```python
from build123d import *

# Parameters (mm, degrees)
SKETCH_W     = 50
SKETCH_H     = 50
PAD_DEPTH    = 50
SKETCH001_W  = 45
SKETCH001_H  = 45
POCKET_DEPTH = 45
FILLET_R     = 2
FILLET001_R  = 2
FILLET002_R  = 2
FILLET003_R  = 2


with BuildPart() as part:
    # Sketch → Pad (new body)
    with BuildSketch(Plane.XY):
        Rectangle(SKETCH_W, SKETCH_H)
    extrude(amount=PAD_DEPTH)

    # Sketch001 (on Face6 of Pad) → Pocket (cut)
    with BuildSketch(Plane.XY.offset(50)):
        Rectangle(SKETCH001_W, SKETCH001_H)
    extrude(amount=-POCKET_DEPTH, mode=Mode.SUBTRACT)

    # Fillet
    fillet_edges = [part.edges().sort_by_distance(p)[0] for p in [
        (25, -25, 25),
    ]]
    fillet(fillet_edges, radius=FILLET_R)

    # Fillet001
    fillet001_edges = [part.edges().sort_by_distance(p)[0] for p in [
        (-25, -25, 25),
    ]]
    fillet(fillet001_edges, radius=FILLET001_R)

    # Fillet002
    fillet002_edges = [part.edges().sort_by_distance(p)[0] for p in [
        (-25, 25, 25),
    ]]
    fillet(fillet002_edges, radius=FILLET002_R)

    # Fillet003
    fillet003_edges = [part.edges().sort_by_distance(p)[0] for p in [
        (25, 25, 25),
    ]]
    fillet(fillet003_edges, radius=FILLET003_R)


solid = part.part
```
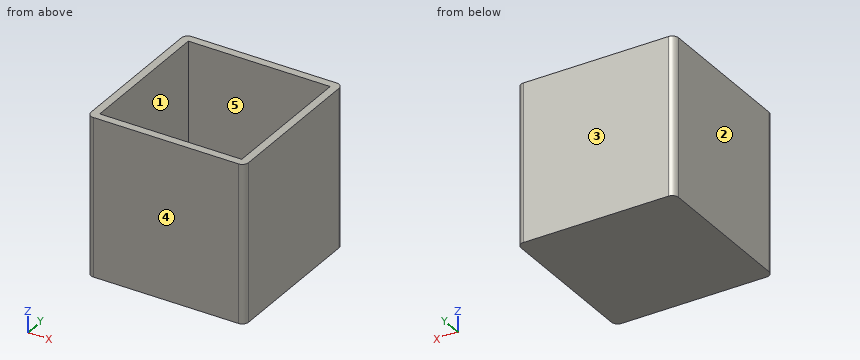
Design review of the part built by this model. Coordinates are the model's own, in mm. Face numbers are marked on the shaded views. A direction names the side the tool comes from. Give positions to 0.01 mm unless a question says otherwise; leave off trailing zeros. Loops run counter-clockwise (first coordinate to the right, second up) from the corner with the lowest first, then second, coordinate; pieces in that order, holes last. Notation, with made-up numbers: M 78.5,-0.5 L 124.5,-0.5 A17 cw 124.5,3.5 Z; hole C -29,53 d7. An arc over 180 degrees is marked long. Return JSON: item names as keys, results as strings. Group by question number.
Item 1: We need section A-A (z = 27). Give the boundary of the cut face in (x, y).
Item 2: Mouldability with a two-part tool opening along Y and no side actions: class the marked faces 1, 2 and 3 as released by +Y, released by -Y, zero draft, split by the parting line, or undercut.
Item 3: We need section B-B (y = -13). Give the boundary of the cut face in (x, z).
Item 4: For probe 1 along Y at (x, z) = (12.5, 20.5); probe 2 along Z at (x, y) = (-2, 13), list the stretches that pass through material, from the lowest coordinate up.
Item 5: Tool access review of the marked faces 4 and 5: name each direction out of +Z, -Z, +X, -X, +Y, -Y from which nothing blocks a thin tool from reaching the whole face with its end or side.
Output:
{
 "1": {"outline": "M -25,-23 A2 ccw -23,-25 L 23,-25 A2 ccw 25,-23 L 25,23 A2 ccw 23,25 L -23,25 A2 ccw -25,23 Z; hole M -22.5,-22.5 L 22.5,-22.5 L 22.5,22.5 L -22.5,22.5 Z"},
 "2": {"face 1": "undercut", "face 2": "zero draft", "face 3": "released by +Y"},
 "3": {"outline": "M -25,0 L 25,0 L 25,50 L 22.5,50 L 22.5,5 L -22.5,5 L -22.5,50 L -25,50 Z"},
 "4": {"probe 1": "y = -25 to -22.5, 22.5 to 25", "probe 2": "z = 0 to 5"},
 "5": {"face 4": "+Z, -Z, +X, -X, -Y", "face 5": "+Z"}
}
